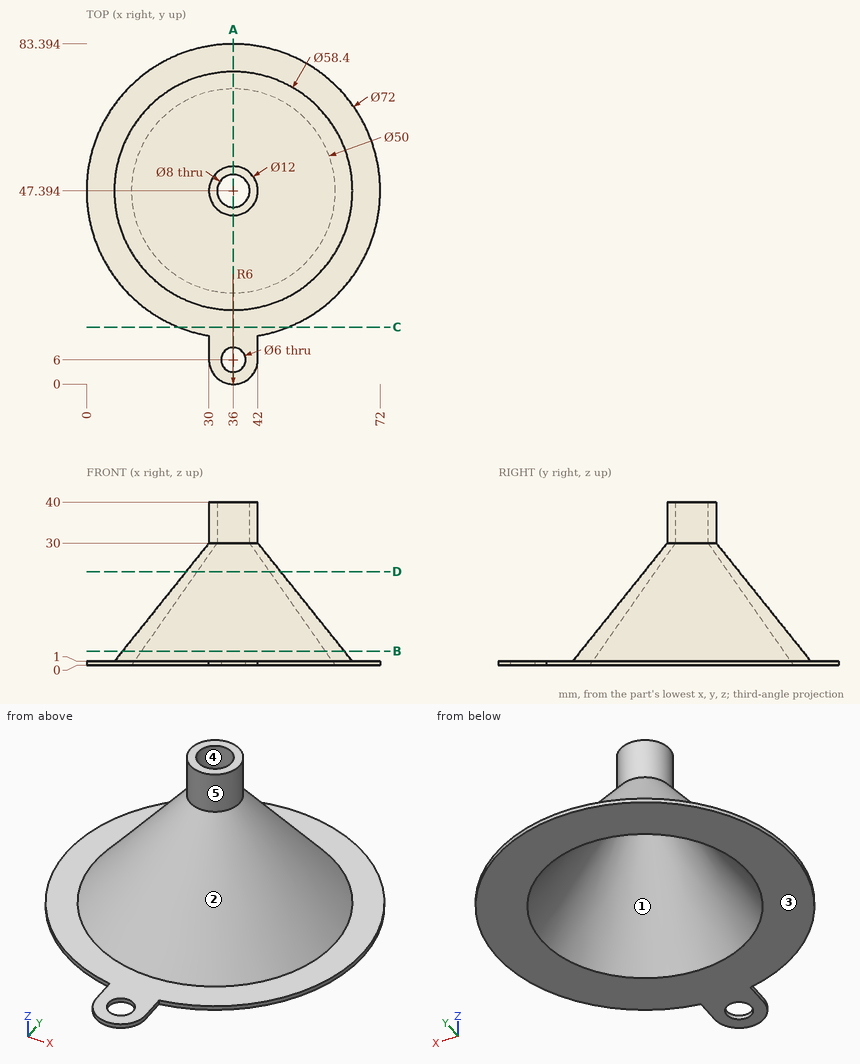
The figure shows three views and two pictorial views of one solid part (mm, origin at its lowest corner). Answer the questions. A direction names the side the tool comes from. Round coordinates to 2 decimals unless told otherwise and drop trailing zeros. Loops run counter-clockwise (first coordinate to the right, second up) from the corner with the lowest first, then second, coordinate; pieces in that order, holes last. Notation, with made-up numbers: M 76,79.25 L 85,79.25 A22 ccw 85,106.25 Z; hole C 52,17 d4. An arc over 180 degrees is marked long. Return JSON: item names as keys, results as strings.
Q1. Each of these flat-tipped pins is pushed along its axis until it touches: pin 1 Ø8 at (y, z) = (54, 5.5) entering from -X; pin 2 Ø7 at (x, y) = (36, 6) entering from -Z; pin 3 Ø12 at (x, y) = (35, 70.5) entering from +Z; pin 4 Ø1 at (y, z) = (43, 30) entering from -X (1 decimal). Where does it stop, or does it pass through?
Results list:
{"pin 1": "stops at x = 7.85", "pin 2": "stops at z = 0", "pin 3": "stops at z = 16.09", "pin 4": "stops at x = 31.2"}
Q2. The mould has two halves that part along Y. Classify the marked faces 1, 2 and 3: released by +Y, released by -Y, zero draft, split by the parting line, or undercut.
Results list:
{"face 1": "undercut", "face 2": "split by the parting line", "face 3": "zero draft"}
Q3. Find section C-C, the plane y = 14. Determine the outline of the cut face in (x, z).
Results list:
{"outline": "M 22.55,0 L 49.45,0 L 49.45,1 L 22.55,1 Z"}
Q4. Which of the six approach directions +Z, -Z, +X, -X, +Y, -Y give full straight-line access (tool end or side, diameter ignored) to the marked faces 4 and 5?
Results list:
{"face 4": "+Z, -Z", "face 5": "+Z"}
Q5. Find section D-D, the plane z = 23. Determine the outline of the cut face in (x, y), plus the area to 3 significant figures.
Results list:
{"outline": "C 36,47.39 d23.2; hole C 36,47.39 d17.8", "area": "174 mm2"}
Q6. Find section A-A, the plane x = 36. Determine the outline of the cut face in (y, z).
Results list:
{"outline": "M 0,0 L 3,0 L 3,1 L 0,1 Z; M 9,0 L 22.39,0 L 43.39,30 L 43.39,40 L 41.39,40 L 41.39,30 L 18.19,1 L 9,1 Z; M 51.39,30 L 72.39,0 L 83.39,0 L 83.39,1 L 76.59,1 L 53.39,30 L 53.39,40 L 51.39,40 Z"}
Q7. Find the intervals of material crossed by line 1 along Y through (x, z) = (36, 0.4); line 2 along Y through (x, z) = (36, 33.75); line 3 along Z through (x, y) = (59.5, 30), in increasing order. Write a range as from..to.
Results list:
{"line 1": "y = 0..3, 9..22.67, 72.11..83.39", "line 2": "y = 41.39..43.39, 51.39..53.39", "line 3": "z = 0..1"}
Q8. Find section B-B, the plane z = 3.5. Determine the outline of the cut face in (x, y).
Results list:
{"outline": "C 36,47.39 d54.4; hole C 36,47.39 d45.1"}
